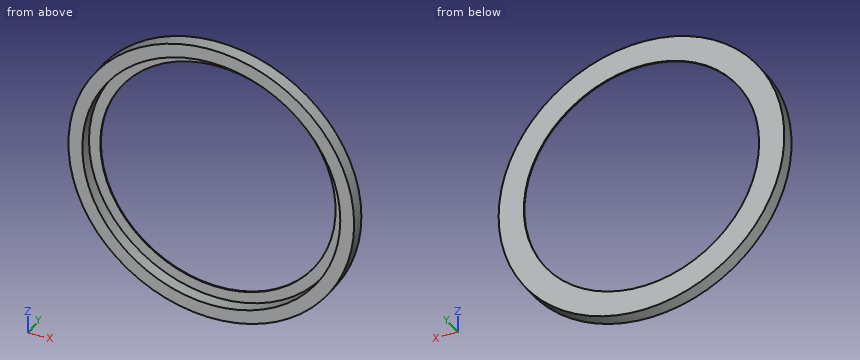
```python
from build123d import *

# Parameters (mm, degrees)
F0_R     = 51
F0_R_2   = 46.05
F1_DEPTH = 5
F2_DEPTH = 0.4
F3_D     = 84


with BuildPart() as f1:
    # F0 (on Front) → F1 (new body)
    with BuildSketch(Plane.XZ):
        Circle(F0_R)
        Circle(F0_R_2, mode=Mode.SUBTRACT)
    extrude(amount=F1_DEPTH)

    # F0 (on Front) → F2 (join)
    with BuildSketch(Plane.XZ):
        Circle(F0_R_2)
    extrude(amount=F2_DEPTH)

    # F3 (through all)
    with Locations(Plane(origin=(0, 0, 0), x_dir=(1, 0, 0), z_dir=(0, 1, 0))):
        with Locations((0, 0)):
            Hole(F3_D / 2)


solid = f1.part
```
CAD build for the part. Positions are in the model's coordinates, mm. Round coordinates to 2 decimals unless told otherwise and drop trailing zeros. Order: outer loops, then holes, each group sorted by start corner. A loop starts at its lowest first (then second) coordinate and runs counter-clockwise, first axis right, second up. Notation, with made-up numbers: (-20, 18.5) -> (-5, 18.5) arc R34 ccw to (-5, 55.5) -> close; hole circle Ø8 at (-28.5, -25.5). An arc over 180 degrees is marked (long way). One line per question, with ' | ' between items.
Q1. Slice it at B-B (x = 0). Write the cut outline in (y, z).
Completed:
outline: (-5, -51) -> (0, -51) -> (0, -42) -> (-0.4, -42) -> (-0.4, -46.05) -> (-5, -46.05) -> close; (-5, 46.05) -> (-0.4, 46.05) -> (-0.4, 42) -> (0, 42) -> (0, 51) -> (-5, 51) -> close
Q2. Probe probe 1 along Z at (x, y) = (0, -3.6); probe 2 along Z at (x, y) = (0, -0.2); probe 3 along Y at (x, z) = (37, 27). List the from-to ranges inside material, lowest first.
Completed:
probe 1: z = -51 to -46.05, 46.05 to 51 | probe 2: z = -51 to -42, 42 to 51 | probe 3: y = -0.4 to 0
Q3. Drop flat-ended pins along their axis: pin 1 (1.5 mm diameter, centred on y = -0.5, z = -4, fed in from +X); pin 2 (1 mm diameter, centred on y = -4, z = -16, fed in from -X). Give the stop position or say it passes through.
Completed:
pin 1: stops at x = 50.9 | pin 2: stops at x = -48.59
Q4. Slice it at C-C (y = -1.95). Write the cut outline in (x, z).
Completed:
outline: circle Ø102 at (0, 0); hole circle Ø92.1 at (0, 0)
Q5. Slice it at A-A (z = 0). Write the cut outline in (x, y), then the cut area to 3 significant figures.
Completed:
outline: (-51, -5) -> (-46.05, -5) -> (-46.05, -0.4) -> (-42, -0.4) -> (-42, 0) -> (-51, 0) -> close; (42, -0.4) -> (46.05, -0.4) -> (46.05, -5) -> (51, -5) -> (51, 0) -> (42, 0) -> close | area: 52.7 mm^2
